Can you work these out from the model? Positions are in its coordinate system, mm. A direction names the side the tool comes from. Give positions to 0.01 mm unless a question says otherwise; leave off trailing zeros. Loops run counter-clockwise (first coordinate to the right, second up) from the corner with the lowest first, then second, coordinate; pieces in that order, holes last. Notation, with made-up numbers: M 51,28 L 93,28 A35 ccw 93,63 Z; hole C -26.5,18.25 d7. An arc over 180 degrees is marked long. Answer as a JSON object with one key per item and string values.
```python
from build123d import *

# Parameters (mm, degrees)
SCHIZZO1_R                   = 10.5
ESTRUSIONE_ESTRUSIONE1_DEPTH = 10.77
ESTRUSIONE_ESTRUSIONE2_START = 10.77
ESTRUSIONE_ESTRUSIONE2_DEPTH = 3
ESTRUSIONE_ESTRUSIONE3_START = -3
SCHIZZO4_W                   = 70
SCHIZZO4_H                   = 27
ESTRUSIONE_ESTRUSIONE3_DEPTH = 21.54


with BuildPart() as part:
    # Schizzo1 → Estrusione-Estrusione1 (new, symmetric)
    with BuildSketch(Plane(origin=(0, 0, 0), x_dir=(0, 0, -1), z_dir=(1, 0, 0))):
        Circle(SCHIZZO1_R)
    extrude(amount=ESTRUSIONE_ESTRUSIONE1_DEPTH, both=True)

    # Schizzo3 → Estrusione-Estrusione2 (add)
    with BuildSketch(Plane(origin=(0, 0, 0), x_dir=(0, 0, -1), z_dir=(1, 0, 0)).offset(ESTRUSIONE_ESTRUSIONE2_START)):
        with BuildLine():
            Line((-100, 13.5), (0, 13.5))
            ThreePointArc((0, 13.5), (13.5, 0), (0, -13.5))
            Line((0, -13.5), (-100, -13.5))
            ThreePointArc((-100, -13.5), (-113.5, 0), (-100, 13.5))
        make_face()
    estrusione_estrusione2 = extrude(amount=ESTRUSIONE_ESTRUSIONE2_DEPTH)

    # Specchia4: Estrusione-Estrusione2 across plane
    add(estrusione_estrusione2.mirror(Plane(origin=(0, 0, 0), x_dir=(0, 0, 1), z_dir=(1, 0, 0))))

    # Schizzo4 → Estrusione-Estrusione3 (add)
    with BuildSketch(Plane(origin=(13.77, 0, 0), x_dir=(0, 0, -1), z_dir=(1, 0, 0)).offset(ESTRUSIONE_ESTRUSIONE3_START)):
        with Locations((-50, 0)):
            Rectangle(SCHIZZO4_W, SCHIZZO4_H)
    extrude(amount=-ESTRUSIONE_ESTRUSIONE3_DEPTH)


solid = part.part
```
1) Suppose I cut it at C-C, the plane z = 8. Write out the boundary of the cut face in (x, y), and give its area (3 significant figures).
Answer list:
{"outline": "M -13.77,-13.5 L -10.77,-13.5 L -10.77,-6.8 L 10.77,-6.8 L 10.77,-13.5 L 13.77,-13.5 L 13.77,13.5 L 10.77,13.5 L 10.77,6.8 L -10.77,6.8 L -10.77,13.5 L -13.77,13.5 Z", "area": "455 mm^2"}
2) For faces 5 (the flat face through (-10.77, 0, 99)), 6 (the flat face through (10.77, -6, 10)), 7 (the cylindrical face through (12.249, -0.297, 113.497)), which set-ups out of +Z, -Z, +X, -X, +Y, -Y let a thin tool reach every point of the face, with its end or its side?
Answer list:
{"face 5": "+Z, +Y, -Y", "face 6": "none", "face 7": "+Z, +X, -X"}
3) Will these pins go through, and if not, where does the flat tip stop? pin 1 Ø8 at (x, y) = (-6.5, -5) entering from +Z; pin 2 Ø12 at (x, y) = (7.5, 3) entering from -Z.
Answer list:
{"pin 1": "z = 85", "pin 2": "z = -13.5"}
4) Suppose I cut it at B-B, the plane x = -4.5. Write out the boundary of the cut face in (y, z), and give its area (3 significant figures).
Answer list:
{"outline": "M -13.5,15 L 13.5,15 L 13.5,85 L -13.5,85 Z; C 0,0 d21", "area": "2,240 mm^2"}
5) If we mould it in two halves opening along Z, with no side actions, what happens to faces 1 (the flat face through (-10.77, -6, 10)), 2 (the flat face through (0, 0, 15)), 3 (the flat face through (0, 0, 85)), 4 (the flat face through (0, -13.5, 49))? For each: +Z half, -Z half, draft (parallel to the pull), parting line (faces both ways), or undercut.
Answer list:
{"face 1": "undercut", "face 2": "undercut", "face 3": "+Z half", "face 4": "draft"}
6) Suppose I cut it at A-A, the plane y = 0. Write out the boundary of the cut face in (x, z), and give its area (3 significant figures).
Answer list:
{"outline": "M -13.77,-13.5 L -10.77,-13.5 L -10.77,-10.5 L 10.77,-10.5 L 10.77,-13.5 L 13.77,-13.5 L 13.77,113.5 L 10.77,113.5 L 10.77,85 L -10.77,85 L -10.77,113.5 L -13.77,113.5 Z; hole M -10.77,10.5 L 10.77,10.5 L 10.77,15 L -10.77,15 Z", "area": "2,720 mm^2"}
7) Please list where these lines run through material, in increasing order: line 1 along X through (y, z) = (-4.25, 14); line 2 along Z through (x, y) = (-0.5, -7.25); line 3 along Z through (x, y) = (-7.5, 9.75). Write a range as from..to.
Answer list:
{"line 1": "-13.77..-10.77, 10.77..13.77", "line 2": "-7.6..7.6, 15..85", "line 3": "-3.9..3.9, 15..85"}
